For this review, take the finished solid that the model builds, in its own axes (mm). A direction names the side the tool comes from. Coordinates: 2 decimals unless noted, no trailing zeros. Write each loop counter-clockwise with the first axis right and the second up, starting at its lowest first coordinate (ties: lowest second). Pieces come first, ordered by that corner, then holes. Notation, with made-up numbers: (-11, 32.5) -> (2, 32.5) arc R9 ccw to (2, 37.5) -> close; hole circle Ø1 at (66, 26.25). An arc over 180 degrees is marked (long way). Put each result on its own line as item: value. Start each with the question number.
Item 1: Consider section A-A on y = 0. Give the boundary of the cut face in (x, z).
Item 2: To check wall thickness, follow L1, parallel to Y at x = -58.5, z = 18.5; L2, parallel to X at y = -22, z = 58.5; L3, parallel to Z at x = -79, y = 0. State the ranges of each line that lie inside material, in increasing order.
Item 3: Consider section B-B on x = -2. Give the boundary of the cut face in (y, z), and give its area (3 significant figures).
Item 4: Insertion check: P1, Ø6, axis at x = 18, z = 29.5, coming from the +Y side; P2, Ø1.3, axis at x = 12, y = -49.5, coming from the +Z side. Each pin has a flat end and moves straight along its axis. Give the tip position at first contact, or say it passes through.
Item 5: Consider section C-C on y = -20. Give the boundary of the cut face in (x, z), and give its area (3 significant figures).
Item 6: The part is to be moulded in two halves that separate along X. For faces 1 (the flat face through (77.135, -1, 19)), 2 (the flat face through (79.675, -1, 19)), 3 (the flat face through (-1, 50.712, 19)), say which applies: +X half, -X half, draft (parallel to the pull), parting line (faces both ways), or undercut.
Item 7: For faces 4 (the flat face through (-77.135, -1, 19)), 5 (the flat face through (-1, -50.712, 19)), list the 3-axis set-ups (+Z, -Z, +X, -X, +Y, -Y) from which the entire face can be reached by the end or side of a thin tool; tool diameter is ignored.
Item 8: Consider section D-D on z = 52.5. Give the boundary of the cut face in (x, y).
```python
from build123d import *

# Parameters (mm, degrees)
F0_W     = 159.349978
F0_H     = 101.423756
F1_DEPTH = 69.088
F2_T     = -2.54
F3_W     = 63.709832
F3_H     = 88.611978
F4_DEPTH = 101.424755
F5_R     = 17.562361
F6_DEPTH = 159.350978


with BuildPart() as f1:
    # F0 (on Top) → F1 (new body)
    with BuildSketch(Plane.XY):
        Rectangle(F0_W, F0_H)
    extrude(amount=F1_DEPTH)

    # F2
    f2_openings = [f1.faces().sort_by_distance(p)[0] for p in [
        (0, 0, 69.088),
        (0, 0, 0),
    ]]
    offset(amount=F2_T, openings=f2_openings)

    # F3 (on face) → F4 (cut, through all)
    with BuildSketch(Plane.XZ.offset(50.711878)):
        with Locations((0, 69.088)):
            Rectangle(F3_W, F3_H)
    extrude(amount=-F4_DEPTH, mode=Mode.SUBTRACT)

    # F5 (on face) → F6 (cut, through all)
    with BuildSketch(Plane.YZ.offset(79.674989)):
        with Locations((0, 36.715534)):
            Circle(F5_R)
    extrude(amount=-F6_DEPTH, mode=Mode.SUBTRACT)


solid = f1.part
```
Return value:
1. outline: (-79.67, 0) -> (-77.13, 0) -> (-77.13, 19.15) -> (-79.67, 19.15) -> close; (-79.67, 54.28) -> (-77.13, 54.28) -> (-77.13, 69.09) -> (-79.67, 69.09) -> close; (77.13, 0) -> (79.67, 0) -> (79.67, 19.15) -> (77.13, 19.15) -> close; (77.13, 54.28) -> (79.67, 54.28) -> (79.67, 69.09) -> (77.13, 69.09) -> close
2. L1: -50.71 to -48.17, 48.17 to 50.71
2. L2: -79.67 to -77.13, 77.13 to 79.67
2. L3: 0 to 19.15, 54.28 to 69.09
3. outline: (-50.71, 0) -> (-48.17, 0) -> (-48.17, 24.78) -> (-50.71, 24.78) -> close; (48.17, 0) -> (50.71, 0) -> (50.71, 24.78) -> (48.17, 24.78) -> close
3. area: 126 mm^2
4. P1: through
4. P2: z = 24.78
5. outline: (-79.67, 0) -> (-77.13, 0) -> (-77.13, 69.09) -> (-79.67, 69.09) -> close; (77.13, 0) -> (79.67, 0) -> (79.67, 69.09) -> (77.13, 69.09) -> close
5. area: 351 mm^2
6. face 1: undercut
6. face 2: +X half
6. face 3: draft
7. face 4: +Z, -Z
7. face 5: +Z, -Z, +X, -X, -Y
8. outline: (-79.67, -50.71) -> (-31.85, -50.71) -> (-31.85, -48.17) -> (-77.13, -48.17) -> (-77.13, -7.7) -> (-79.67, -7.7) -> close; (-79.67, 7.7) -> (-77.13, 7.7) -> (-77.13, 48.17) -> (-31.85, 48.17) -> (-31.85, 50.71) -> (-79.67, 50.71) -> close; (31.85, -50.71) -> (79.67, -50.71) -> (79.67, -7.7) -> (77.13, -7.7) -> (77.13, -48.17) -> (31.85, -48.17) -> close; (31.85, 48.17) -> (77.13, 48.17) -> (77.13, 7.7) -> (79.67, 7.7) -> (79.67, 50.71) -> (31.85, 50.71) -> close
